Geometry: final body of the model. Coordinates: model frame, mm. A direction names the side the tool comes from. Coordinates: 2 decimals unless noted, no trailing zeros. Order: outer loops, then holes, each group sorted by start corner. A loop starts at its lowest first (then second) coordinate and runs counter-clockwise, first axis right, second up. Notation, with made-up numbers: M 28,19.25 L 77,19.25 A12 ccw 77,32.25 Z; hole C 44.25,65.25 d10. An arc over 180 degrees is marked long. Use CSV: the item, a comma, the result in double quotes. Start each with the question number.
Q1. Section query D-D, the plane x = 16. Output: boundary loops of the cut face in (y, z), and give its area (3 significant figures).
Q2. Section query C-C, the plane z = 3.25. State how many separate pieces and enclosed holes the cut face has, and give its area (3 significant figures).
Q3. Access query for faces 5 (the face through (14, -19.297, 2)), 6 (the face through (-5, 7.703, 2)), 7 (the face through (-16, -26.297, 2)), 8 (the face through (28.413, -9.077, 2.465)). Directions: +Z, -Z, +X, -X, +Y, -Y. A direction counts if a zero-diameter tool reaches every point of the face in a straight line with its end or side. Return the directions, or none.
Q4. Section query B-B, the plane y = -22. Output: boundary loops of the cut face in (x, z), and give its area (3 significant figures).
Q5. Mould query, pull axis X, two halves, no side actions, for faces 1 (the face through (17.74, -1.62, 2.46)), 2 (the face through (-9.82, -30.22, 2.46)), 3 (the face through (-5.845, -28, 2)), 4 (the face through (-1, -10, 0)). Classes: +X half, -X half, draft (parallel to the pull), parting line (faces both ways), or undercut.
Q6. First-contact query: P1, Ø1, axis at x = 9, z = 1, coming from the -Y side; P2, Ø1.8, axis at x = -9.08, y = 4.2, coming from the -Z side; P3, Ø3, axis at y = 1, z = 2.5, coming from the +X side; P4, Ø2, axis at x = -1, z = 1, coming from the +Y side. Flat tips, straight axial feed; report the tip coordinate or a pass-through.
Q7. Ray query, probe 1 along Y at (x, z) = (18.5, 2); probe 2 along Y at (x, z) = (-9.5, 3.65); probe 3 along Y at (x, z) = (18, 3.55). Return the intervals inside material, ascending.
Q8. Section query A-A, the plane x = 25.5. Output: boundary loops of the cut face in (y, z), and give its area (3 significant figures).
from build123d import *

# Parameters (mm, degrees)
ESQUISSE1_R             = 1
ESQUISSE1_R_2           = 1.5
BOSS_EXTRU_1_DEPTH      = 5
ENL_V_MAT_EXTRU_1_DEPTH = 5
ESQUISSE3_W             = 20
ESQUISSE3_H             = 34
BOSS_EXTRU_2_DEPTH      = 5
ESQUISSE4_R             = 1.5
ESQUISSE4_W             = 9.798464728
ESQUISSE4_H             = 39.858161606
ENL_V_MAT_EXTRU_2_DEPTH = 5
ESQUISSE5_W             = 2.5
ESQUISSE5_H             = 34
BOSS_EXTRU_3_DEPTH      = 5
ESQUISSE6_R             = 1.6
BOSS_EXTRU_4_DEPTH      = 5
CONG_1_R                = 10
CONG_2_R                = 10


with BuildPart() as part:
    # Esquisse1 → Boss.-Extru.1 (new body)
    with BuildSketch(Plane.XY):
        with BuildLine():
            Line((-13.584596858, -30.047129187), (-13.584596858, -25.547129187))
            Line((-13.584596858, -25.547129187), (-13.584596858, -25.297129187))
            Line((-13.584596858, -25.297129187), (-13.834596858, -25.297129187))
            Line((-13.834596858, -25.297129187), (-16.334596858, -25.297129187))
            Line((-16.334596858, -25.297129187), (-16.584596858, -25.297129187))
            Line((-16.584596858, -25.297129187), (-16.584596858, -25.047129187))
            Line((-16.584596858, -25.047129187), (-16.584596858, 6.452870813))
            Line((-16.584596858, 6.452870813), (-16.584596858, 6.702870813))
            Line((-16.584596858, 6.702870813), (-16.334596858, 6.702870813))
            Line((-16.334596858, 6.702870813), (-13.834596858, 6.702870813))
            Line((-13.834596858, 6.702870813), (-13.584596858, 6.702870813))
            Line((-13.584596858, 6.702870813), (-13.584596858, 6.952870813))
            Line((-13.584596858, 6.952870813), (-13.584596858, 11.452870813))
            Line((-13.584596858, 11.452870813), (-13.584596858, 11.702870813))
            Line((-13.584596858, 11.702870813), (-13.334596858, 11.702870813))
            Line((-13.334596858, 11.702870813), (-8.584596858, 11.702870813))
            Line((-8.584596858, 11.702870813), (-8.584596858, 6.702870813))
            Line((-8.584596858, 6.702870813), (-7.491776281, 6.702870813))
            Line((-7.491776281, 6.702870813), (-4.034541178, 6.702870813))
            ThreePointArc((-4.034541178, 6.702870813), (-0.161557832, 6.19424756), (3.448773595, 4.702870813))
            ThreePointArc((3.448773595, 4.702870813), (10.66943645, 1.720117321), (18.415403142, 0.702870813))
            ThreePointArc((18.415403142, 0.702870813), (28.415403142, -9.297129187), (18.415403142, -19.297129187))
            ThreePointArc((18.415403142, -19.297129187), (10.66943645, -20.314375694), (3.448773595, -23.297129187))
            ThreePointArc((3.448773595, -23.297129187), (-0.161557832, -24.788505933), (-4.034541178, -25.297129187))
            Line((-4.034541178, -25.297129187), (-7.491776281, -25.297129187))
            Line((-7.491776281, -25.297129187), (-8.584596858, -25.297129187))
            Line((-8.584596858, -25.297129187), (-8.584596858, -30.297129187))
            Line((-8.584596858, -30.297129187), (-13.334596858, -30.297129187))
            Line((-13.334596858, -30.297129187), (-13.584596858, -30.297129187))
            Line((-13.584596858, -30.297129187), (-13.584596858, -30.047129187))
        make_face()
        with Locations((18.477857718, -2.297129187)):
            Circle(ESQUISSE1_R, mode=Mode.SUBTRACT)
        with Locations((25.415403142, -9.359583762)):
            Circle(ESQUISSE1_R, mode=Mode.SUBTRACT)
        with Locations((18.415403142, -9.297129187)):
            Circle(ESQUISSE1_R_2, mode=Mode.SUBTRACT)
        with Locations((11.415403142, -9.234674611)):
            Circle(ESQUISSE1_R, mode=Mode.SUBTRACT)
        with Locations((18.352948567, -16.297129187)):
            Circle(ESQUISSE1_R, mode=Mode.SUBTRACT)
    extrude(amount=BOSS_EXTRU_1_DEPTH)

    # Esquisse2 → Enlèv. mat.-Extru.1 (cut)
    with BuildSketch(Plane(origin=(0, 0, 0), x_dir=(-1, 0, 0), z_dir=(0, 0, -1))):
        Polygon((1.584596858, -19.297129187), (1.584596858, -25.297129187), (1.584596858, -26.297129187), (21.584596858, -26.297129187), (21.584596858, -33.65697819), (-26.833247513, -33.65697819), (-26.198667142, -19.297129187), align=None)
        Polygon((21.584596858, 7.702870813), (1.584596858, 7.702870813), (1.584596858, 6.702870813), (1.584596858, 0.702870813), (-26.198667142, 0.702870813), (-26.833247513, 15.062719816), (21.584596858, 15.062719816), align=None)
    extrude(amount=-ENL_V_MAT_EXTRU_1_DEPTH, mode=Mode.SUBTRACT)

    # Esquisse3 → Boss.-Extru.2 (add)
    with BuildSketch(Plane(origin=(0, 0, 0), x_dir=(-1, 0, 0), z_dir=(0, 0, -1))):
        with Locations((11.584596858, -9.297129187)):
            Rectangle(ESQUISSE3_W, ESQUISSE3_H)
    extrude(amount=-BOSS_EXTRU_2_DEPTH)

    # Esquisse4 → Enlèv. mat.-Extru.2 (cut)
    with BuildSketch(Plane(origin=(0, 0, 0), x_dir=(-1, 0, 0), z_dir=(0, 0, -1))):
        with Locations((9.084596858, -22.797129187)):
            Circle(ESQUISSE4_R)
        with Locations((9.084596858, 4.202870813)):
            Circle(ESQUISSE4_R)
        with Locations((23.983829222, -9.020336398)):
            Rectangle(ESQUISSE4_W, ESQUISSE4_H)
    extrude(amount=-ENL_V_MAT_EXTRU_2_DEPTH, mode=Mode.SUBTRACT)

    # Esquisse5 → Boss.-Extru.3 (add)
    with BuildSketch(Plane(origin=(0, 0, 0), x_dir=(-1, 0, 0), z_dir=(0, 0, -1))):
        with Locations((0.334596858, -9.297129187)):
            Rectangle(ESQUISSE5_W, ESQUISSE5_H)
    extrude(amount=-BOSS_EXTRU_3_DEPTH)

    # Esquisse6 → Boss.-Extru.4 (add)
    # profile 1 of 2: a face of its own
    with BuildSketch(Plane(origin=(0, 0, 0), x_dir=(-1, 0, 0), z_dir=(0, 0, -1))):
        with BuildLine():
            Line((12.324596858, -25.12480516), (5.844596858, -25.12480516))
            Line((5.844596858, -25.12480516), (5.844596858, -28.797129187))
            ThreePointArc((5.844596858, -28.797129187), (9.084596858, -32.037129187), (12.324596858, -28.797129187))
            Line((12.324596858, -28.797129187), (12.324596858, -25.12480516))
        make_face()
        with Locations((9.084596858, -28.797129187)):
            Circle(ESQUISSE6_R, mode=Mode.SUBTRACT)
    # profile 2 of 2: a face of its own
    with BuildSketch(Plane(origin=(0, 0, 0), x_dir=(-1, 0, 0), z_dir=(0, 0, -1))):
        with BuildLine():
            Line((12.324596858, 6.757738308), (5.844596858, 6.757738308))
            Line((5.844596858, 6.757738308), (5.844596858, 10.202870813))
            ThreePointArc((5.844596858, 10.202870813), (9.084596858, 13.442870813), (12.324596858, 10.202870813))
            Line((12.324596858, 10.202870813), (12.324596858, 6.757738308))
        make_face()
        with Locations((9.084596858, 10.202870813)):
            Circle(ESQUISSE6_R, mode=Mode.SUBTRACT)
    extrude(amount=-BOSS_EXTRU_4_DEPTH)

    # Congé1
    # the kernel refuses this fillet: 10 mm, written as the material it adds along each edge
    with BuildSketch(Plane(origin=(0.915403142, 0.702870813, 0), x_dir=(1, 0, 0), z_dir=(0, 0, 1))) as cong_1_piece_1:
        with BuildLine():
            CenterArc((9.539392014, 10), CONG_1_R, 197.457603124, 72.542396876)
            Line((0, 7), (-0.19078784, 6.94))
            ThreePointArc((-0.19078784, 6.94), (-0.2, 3.5), (-0.2, 0))
            Line((-0.2, 0), (0, -0.2))
            Line((0, -0.2), (9.539392014, -0.2))
            Line((9.539392014, -0.2), (9.539392014, 0))
        make_face()
    extrude(amount=5)
    with BuildSketch(Plane(origin=(0.915403142, -19.297129187, 5), x_dir=(0, -1, 0), z_dir=(0, 0, -1))) as cong_1_piece_2:
        with BuildLine():
            CenterArc((10, -9.539392014), CONG_1_R, 107.457603124, 72.542396876)
            Line((0, -9.539392014), (-0.2, -9.539392014))
            Line((-0.2, -9.539392014), (-0.2, 0))
            Line((-0.2, 0), (0, 0.2))
            ThreePointArc((0, 0.2), (3.5, 0.2), (6.94, 0.19078784))
            Line((6.94, 0.19078784), (7, 0))
        make_face()
    extrude(amount=5)

    # Congé2
    cong_2_edges = [part.edges().sort_by_distance(p)[0] for p in [
        (0.915403142, -26.297129187, 2.5),
        (0.915403142, 7.702870813, 2.5),
    ]]
    fillet(cong_2_edges, radius=CONG_2_R)


solid = part.part
Responses:
1,outline,"M -19.3,0 L 0.7,0 L 0.7,5 L -19.3,5 Z"
1,area,"100 mm²"
2,separate pieces,"1"
2,enclosed holes,"9"
2,area,"1,230 mm²"
3,face 5,"+Z, -Z, +X, -Y"
3,face 6,"+Z, -Z, +X, +Y"
3,face 7,"+Z, -Z, -X, -Y"
3,face 8,"+Z, -Z, +X"
4,outline,"M -19.08,0 L -10.36,0 L -10.36,5 L -19.08,5 Z; M -7.81,0 L 3.62,0 L 3.62,5 L -7.81,5 Z"
4,area,"101 mm²"
5,face 1,"undercut"
5,face 2,"undercut"
5,face 3,"+X half"
5,face 4,"draft"
6,P1,"stops at y = -19.49"
6,P2,"passes through"
6,P3,"stops at x = 23.17"
6,P4,"stops at y = 7.32"
7,probe 1,"y = -19.3 to -17.29, -15.31 to -10.79, -7.8 to -3.3, -1.3 to 0.7"
7,probe 2,"y = -32.01 to -30.34, -27.25 to -24.24, -21.36 to 2.76, 5.64 to 8.66, 11.75 to 13.42"
7,probe 3,"y = -19.3 to -17.23, -15.36 to -10.74, -7.86 to -3.18, -1.42 to 0.7"
8,outline,"M -16.35,0 L -10.36,0 L -10.36,5 L -16.35,5 Z; M -8.36,0 L -2.24,0 L -2.24,5 L -8.36,5 Z"
8,area,"60.6 mm²"
